Can you work these out from the model? Positions are in its coordinate system, mm. Face numbers are marked on the shaded views. A direction names the side the tool comes from. Round coordinates to 2 decimals unless told otherwise and drop trailing zeros. Loops run counter-clockwise (first coordinate to the right, second up) from the corner with the lowest first, then second, coordinate; pieces in that order, holes last.
(1) Thinking about a two-plate mould opening in Y: for the marked faces 1, 2 and 3, which applies, released by +Y, released by -Y, zero draft, split by the parting line, or undercut?
(2) I want a section at B-B on y = -11.75. Write out the boundary of the cut face in (x, z).
(3) Will these pins go through, and if not, where does the flat tip stop? pin 1 Ø2.5 at (y, z) = (-18.5, 3) entering from +X; pin 2 Ø2.5 at (y, z) = (-16.5, 1.5) entering from -X.
(4) I want a section at A-A on z = 2.9. Write out the boundary of the cut face in (x, y).
(5) I want a section at D-D on z = 1.35. Write out the boundary of the cut face in (x, y).
(6) Which directions (+Z, -Z, +X, -X, +Y, -Y) give clear straight access to the entire face, cutting with the end or side of a thin tool? Please do the marked faces 4 and 5.
(7) If I drill on line 1 along Y through (x, z) = (-156.5, 4.2); line 2 along X through (y, z) = (-8.5, 4.6); line 3 along Y through (x, z) = (-143.75, 3.2), over which ranges is the centre line in solid material (lowest first)?
(8) I want a section at C-C on x = -155.75. Write out the boundary of the cut face in (y, z).
from build123d import *

# Parameters (mm, degrees)
SKETCH1_R           = 1.6
BOSS_EXTRUDE1_DEPTH = 5
SKETCH2_R           = 5
CUT_EXTRUDE1_DEPTH  = 162.695924751


with BuildPart() as part:
    # Sketch1 → Boss-Extrude1 (new body)
    with BuildSketch(Plane.XY):
        with BuildLine():
            Line((-154.198398621, -11.402119157), (-154.198398621, -23.477952613))
            Line((-154.198398621, -23.477952613), (-145.198398621, -23.477952613))
            Line((-145.198398621, -23.477952613), (-145.198398621, -11.402119157))
            ThreePointArc((-145.198398621, -11.402119157), (-139.248398621, -8.567952613), (-145.198398621, -5.733786068))
            Line((-145.198398621, -5.733786068), (-145.198398621, -1.727952613))
            Line((-145.198398621, -1.727952613), (-154.198398621, -1.727952613))
            Line((-154.198398621, -1.727952613), (-154.198398621, -5.733786068))
            ThreePointArc((-154.198398621, -5.733786068), (-160.148398621, -8.567952613), (-154.198398621, -11.402119157))
        make_face()
        with Locations((-156.498398621, -8.567952613)):
            Circle(SKETCH1_R, mode=Mode.SUBTRACT)
        with Locations((-142.898398621, -8.567952613)):
            Circle(SKETCH1_R, mode=Mode.SUBTRACT)
    extrude(amount=BOSS_EXTRUDE1_DEPTH)

    # Sketch2 → Cut-Extrude1 (cut, through all)
    with BuildSketch(Plane(origin=(0, -1.727952613, 0), x_dir=(1, 0, 0), z_dir=(0, 1, 0))):
        with Locations((-149.698398621, -7)):
            Circle(SKETCH2_R)
    extrude(amount=-CUT_EXTRUDE1_DEPTH, mode=Mode.SUBTRACT)


solid = part.part
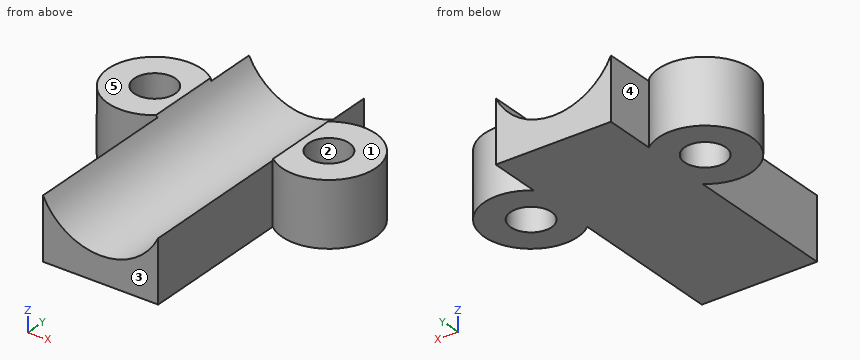
Filled sheet:
1. face 1: zero draft
1. face 2: undercut
1. face 3: released by -Y
2. outline: (-158.29, 0) - (-154.71, 0) - (-154.71, 5) - (-158.29, 5) - close; (-154.2, 0) - (-145.2, 0) - (-145.2, 4.82) arc R5 cw to (-154.2, 4.82) - close; (-144.69, 0) - (-141.11, 0) - (-141.11, 5) - (-144.69, 5) - close
3. pin 1: stops at x = -145.2
3. pin 2: stops at x = -154.2
4. outline: (-154.2, -23.48) - (-152.56, -23.48) - (-152.56, -1.73) - (-154.2, -1.73) - (-154.2, -5.73) arc R3.65 ccw (long way) to (-154.2, -11.4) - close; (-146.84, -23.48) - (-145.2, -23.48) - (-145.2, -11.4) arc R3.65 ccw (long way) to (-145.2, -5.73) - (-145.2, -1.73) - (-146.84, -1.73) - close; hole circle Ø3.2 at (-156.5, -8.57); hole circle Ø3.2 at (-142.9, -8.57)
5. outline: (-154.2, -23.48) - (-145.2, -23.48) - (-145.2, -11.4) arc R3.65 ccw (long way) to (-145.2, -5.73) - (-145.2, -1.73) - (-154.2, -1.73) - (-154.2, -5.73) arc R3.65 ccw (long way) to (-154.2, -11.4) - close; hole circle Ø3.2 at (-156.5, -8.57); hole circle Ø3.2 at (-142.9, -8.57)
6. face 4: +Z, -Z, +Y
6. face 5: +Z, +X, -X, +Y, -Y
7. line 1: y = -12.22 to -10.17, -6.97 to -4.92
7. line 2: x = -160.15 to -158.1, -154.9 to -154.08, -145.31 to -144.5, -141.3 to -139.25
7. line 3: y = -12.12 to -9.92, -7.21 to -5.02
8. outline: (-12.14, 0) - (-9.98, 0) - (-9.98, 5) - (-12.14, 5) - close; (-7.15, 0) - (-5, 0) - (-5, 5) - (-7.15, 5) - close
